Check sheet for the modelled part. Datum: model origin and axes. Units: mm. Round coordinates to 2 decimals unless told otherwise and drop trailing zeros. Loops run counter-clockwise (first coordinate to the right, second up) from the corner with the lowest first, then second, coordinate; pieces in that order, holes last. Notation, with made-up numbers: (43, 17) -> (68, 17) arc R27 ccw to (68, 38) -> close; hole circle Ø4 at (69, 29.25). An arc over 180 degrees is marked (long way). Use one line per item in the form item = value. Start each with the question number.
(1) Go/stop test with flat-tipped pins: pin 1 (5 mm diameter, centred on x = 16, z = 6.5, fed in from +Y); pin 2 (3 mm diameter, centred on x = 19.5, z = 11.5, fed in from -Y). Record where each tip stops, or that it passes through.
(2) Sectioned sample at A-A (z = 17). Record the cut outline in (x, y).
(3) Material ranges on probe 1 along X at (y, z) = (571, 10.5); probe 2 along Y at (x, z) = (25.5, 27.75); probe 3 along Y at (x, z) = (27, 3), recorded low to high. Write a range as [from, to].
(4) Sectioned sample at B-B (x = 24.5). Record the cut outline in (y, z).
from build123d import *

# Parameters (mm, degrees)
SKETCH_1_W          = 30
SKETCH_1_H          = 30
EXTRUDE_1_DEPTH     = 600
CUT_EXTRUDE_1_REACH = 603.498
CUT_EXTRUDE_2_REACH = 603.498
CUT_EXTRUDE_3_DEPTH = 602.498129673
EXTRUDE_2_DEPTH     = 30


with BuildPart() as part:
    # 草图1 → 凸台-拉伸1 (new body)
    with BuildSketch(Plane(origin=(0, 0, 0), x_dir=(1, 0, 0), z_dir=(0, 1, 0))):
        with Locations((15, -15)):
            Rectangle(SKETCH_1_W, SKETCH_1_H)
    extrude(amount=EXTRUDE_1_DEPTH)

    # 草图2 → 切除-拉伸1 (cut, up to next)
    with BuildSketch(Plane.XY.offset(30), mode=Mode.PRIVATE) as cut_extrude_1_sk1:
        Polygon((0, 0), (30, 8.038475773), (30, 0), align=None)
    cut_extrude_1_tool1 = extrude(cut_extrude_1_sk1.sketch, amount=-CUT_EXTRUDE_1_REACH, mode=Mode.PRIVATE) & part.part
    add(cut_extrude_1_tool1.solids().sort_by_distance((20, 2.679492, 30))[0], mode=Mode.SUBTRACT)

    # 草图3 → 切除-拉伸2 (cut, up to next)
    with BuildSketch(Plane(origin=(0, 0, 0), x_dir=(-1, 0, 0), z_dir=(0, 0, -1)), mode=Mode.PRIVATE) as cut_extrude_2_sk1:
        Polygon((0, 600), (-30, 600), (-30, 488.038475773), align=None)
    cut_extrude_2_tool1 = extrude(cut_extrude_2_sk1.sketch, amount=-CUT_EXTRUDE_2_REACH, mode=Mode.PRIVATE) & part.part
    add(cut_extrude_2_tool1.solids().sort_by_distance((20, 562.679492, 0))[0], mode=Mode.SUBTRACT)

    # 草图5 → 切除-拉伸3 (cut, through all)
    with BuildSketch(Plane(origin=(0, 0, 0), x_dir=(-1, 0, 0), z_dir=(0, 0, -1))):
        Polygon((-30, 17.320508076), (-30, 8.038475773), (0, 0), align=None)
    extrude(amount=-CUT_EXTRUDE_3_DEPTH, mode=Mode.SUBTRACT)

    # 草图6 → 凸台-拉伸2 (add)
    with BuildSketch(Plane(origin=(0, 0, 0), x_dir=(-1, 0, 0), z_dir=(0, 0, -1))):
        Polygon((-30, 488.038475773), (0, 600), (-30, 548.038475773), align=None)
    extrude(amount=-EXTRUDE_2_DEPTH)


solid = part.part
Checks:
q1.pin_1 = 576.62
q1.pin_2 = 10.39
q2.outline = (0, 0) -> (30, 17.32) -> (30, 548.04) -> (0, 600) -> close
q3.probe_1 = [0, 16.74]
q3.probe_2 = [14.72, 555.83]
q3.probe_3 = [15.59, 553.23]
q4.outline = (14.15, 0) -> (557.56, 0) -> (557.56, 30) -> (14.15, 30) -> close
